The listing builds one solid part. Answer for the finished solid, in the listing's coordinates (mm). A direction names the side the tool comes from. Round coordinates to 2 decimals unless told otherwise and drop trailing zeros. Write each loop counter-clockwise with the first axis right and the second up, starting at its lowest first coordinate (ties: lowest second). Pieces come first, ordered by that corner, then holes. Notation, with made-up numbers: (46, 2) - (103, 2) arc R25 cw to (103, 23) - close; hole circle Ø1 at (22.25, 48). An arc over 180 degrees is marked (long way). Use a Markdown table: item, result. Add a question column.
1) A cutting plane is placed at B-B (x = 0.75). Give the vertices of the cut face in (y, z), then the cut area to 3 significant figures.
2) A tool of negligible diameter and unlimited length cuts with its end or side. For faces 4 (the flat face through (-13, 0, -18)), 5 (the flat face through (2, 5, -1)), from which of +Z, -Z, +X, -X, +Y, -Y can it reach the whole face along a straight path? Write none if from no direction.
3) Find the intervals of material crossed by probe 1 along Z at (x, y) = (1.75, -2.25); probe 2 along Y at (x, z) = (11.25, -32.5); probe 3 along X at (y, z) = (11, -13), in increasing order. Write a range as from..to.
4) Each of these flat-tipped pins is pushed along its axis until it touches: P1, Ø0.7, axis at x = 5, z = -1, coming from the -Y side; P2, Ø1.1, axis at y = 5, z = -0.5, coming from the +X side. Where does it stop, or does it pass through?
5) A cutting plane is placed at A-A (z = -33). Give the vertices of the cut face in (x, y), then the cut area to 3 significant figures.
6) Determine the mould class of faces 1 (the flat face through (1, -11.118, -1)), 2 (the flat face through (0, 0, -36)), 3 (the cylindrical face through (-0.112, 12.639, -0.342)) for opening direction Y: +Y half, -Y half, draft (parallel to the pull), parting line (faces both ways), or undercut.
```python
from build123d import *

# Parameters (mm, degrees)
F0_W     = 2
F0_H     = 2
F0_H_2   = 9.117820628
F0_W_2   = 4.7262388766
F1_DEPTH = 36
F2_DEPTH = 1.4
F3_R     = 5
F4_R     = 1.2


with BuildPart() as f1:
    # F0 (on Top) → F1 (new body)
    with BuildSketch(Plane.XY):
        Polygon((13, -13), (13, 0), (13, 13), (-13, 13), (-13, -13), align=None)
        Polygon((-10.2526927367, 0), (0, 10.9954001382), (2, 10.9954001382), (2, 0), (6.7262388766, 0), (6.7262388766, -2), (2, -2), (2, -11.117820628), (0, -11.117820628), (0, -2), (-10.2526927367, -2), align=None, mode=Mode.SUBTRACT)
        Polygon((0, 8.8505196818), (0, 10.9954001382), (-10.2526927367, 0), (-8.2526927367, 0), align=None)
        Polygon((-8.2526927367, 0), (-10.2526927367, 0), (-10.2526927367, -2), (0, -2), (0, 0), align=None)
        Polygon((0, 0), (0, 8.8505196818), (-8.2526927367, 0), align=None)
        Polygon((2, 0), (2, 10.9954001382), (0, 8.8505196818), (0, 0), align=None)
        Polygon((2, 10.9954001382), (0, 10.9954001382), (0, 8.8505196818), align=None)
        with Locations((1, -1)):
            Rectangle(F0_W, F0_H)
        with Locations((1, -6.558910314)):
            Rectangle(F0_W, F0_H_2)
        with Locations((4.3631194383, -1)):
            Rectangle(F0_W_2, F0_H)
    extrude(amount=-F1_DEPTH)

    # F0 (on Top) → F2 (cut)
    with BuildSketch(Plane.XY):
        Polygon((0, 8.8505196818), (0, 10.9954001382), (-10.2526927367, 0), (-8.2526927367, 0), align=None)
        Polygon((2, 10.9954001382), (0, 10.9954001382), (0, 8.8505196818), align=None)
        Polygon((2, 0), (2, 10.9954001382), (0, 8.8505196818), (0, 0), align=None)
        with Locations((4.3631194383, -1)):
            Rectangle(F0_W_2, F0_H)
        with Locations((1, -6.558910314)):
            Rectangle(F0_W, F0_H_2)
        with Locations((1, -1)):
            Rectangle(F0_W, F0_H)
        Polygon((-8.2526927367, 0), (-10.2526927367, 0), (-10.2526927367, -2), (0, -2), (0, 0), align=None)
    extrude(amount=-F2_DEPTH, mode=Mode.SUBTRACT)

    # F3
    f3_edges = [f1.edges().sort_by_distance(p)[0] for p in [
        (13, 13, -18),
        (13, -13, -18),
        (-13, -13, -18),
        (-13, 13, -18),
    ]]
    fillet(f3_edges, radius=F3_R)

    # F4
    f4_edges = [f1.edges().sort_by_distance(p)[0] for p in [
        (-13, 0, 0),
        (-11.535534, 11.535534, 0),
        (0, 13, 0),
        (-11.535534, -11.535534, 0),
        (0, -13, 0),
        (11.535534, -11.535534, 0),
        (13, 0, 0),
        (11.535534, 11.535534, 0),
        (13, 0, -36),
        (11.535534, -11.535534, -36),
        (11.535534, 11.535534, -36),
        (0, -13, -36),
        (0, 13, -36),
        (-11.535534, -11.535534, -36),
        (-11.535534, 11.535534, -36),
        (-13, 0, -36),
    ]]
    fillet(f4_edges, radius=F4_R)


solid = f1.part
```
Entries:
| question | item | result |
|---|---|---|
| 1 | outline | (-13, -34.8) arc R1.2 ccw to (-11.8, -36) - (11.8, -36) arc R1.2 ccw to (13, -34.8) - (13, -1.2) arc R1.2 ccw to (11.8, 0) - (11, 0) - (11, -1.4) - (-11.12, -1.4) - (-11.12, 0) - (-11.8, 0) arc R1.2 ccw to (-13, -1.2) - close |
| 1 | area | 904 mm² |
| 2 | face 4 | +Z, -Z, -X, +Y, -Y |
| 2 | face 5 | +Z |
| 3 | probe 1 | z = -36..-1.4 |
| 3 | probe 2 | y = -11.8..11.8 |
| 3 | probe 3 | x = -12..12 |
| 4 | P1 | stops at y = -13 |
| 4 | P2 | stops at x = 12.99 |
| 5 | outline | (-13, -8) arc R5 ccw to (-8, -13) - (8, -13) arc R5 ccw to (13, -8) - (13, 8) arc R5 ccw to (8, 13) - (-8, 13) arc R5 ccw to (-13, 8) - close |
| 5 | area | 655 mm² |
| 6 | face 1 | undercut |
| 6 | face 2 | draft |
| 6 | face 3 | +Y half |
